Design review of the part built by this model. Coordinates are the model's own, in mm. A direction names the side the tool comes from. Round coordinates to 2 decimals unless told otherwise and drop trailing zeros. Order: outer loops, then holes, each group sorted by start corner. A loop starts at its lowest first (then second) coordinate and runs counter-clockwise, first axis right, second up. Notation, with made-up numbers: M 69,47 L 76,47 A10 cw 76,65 Z; hole C 88.25,83.25 d11. An arc over 180 degrees is marked long. Write each question's results on one line, items separated by ' | '. Start each with the question number.
Item 1: Take a section at B-B, the plane x = 14. Write out the cut boundary in (y, z), plus the area to 3 significant figures.
Item 2: The part is to be moulded in two halves that separate along Z. For faces 1 (the cylindrical face through (-38.356, 14.529, -14.345)), 2 (the cylindrical face through (101.339, -33.056, -8.385)), 3 (the flat face through (-23, 8, -18.019)), 4 (the flat face through (25, -3, 0)), say which applies: +Z half, -Z half, draft (parallel to the pull), parting line (faces both ways), or undercut.
Item 3: Take a section at A-A, the plane z = 3.5. Write out the cut boundary in (x, y).
Item 4: Machinability: for faces 5 (the flat face through (94.126, -28.892, -9.07)), 6 (the flat face through (24, -4.5, -9)), 7 (the flat face through (79.126, -20.232, -8.93)), which of the approach directions +Z, -Z, +X, -X, +Y, -Y give a long, thin tool a straight path to every point of the face, cutting with its end or side? Answer none if there is none.
Item 5: Clearance check with flat-ended pins moving along their axes: pin 1 (0.6 mm diameter, centred on x = 27, z = -16.5, fed in from +Y); pin 2 (10 mm diameter, centred on y = -12.5, z = 1.5, fed in from -X); pin 3 (7 mm diameter, centred on x = 22.5, z = -8.5, fed in from +Y); pin 4 (9 mm diameter, centred on x = 12, y = -12, fed in from -Z). State where each tip first meets the part, or that it passes through.
Item 6: Wall thickness on line 1 (Z direction, x = -11.5, y = 3); line 2 (Y direction, x = 45.5, z = -4); line 3 (X direction, y = 7, z = -15): over which ranges is each line inside the solid? List them lowest first. Write a range as [from, to].
Item 7: Take a section at C-C, the plane y = -7.5. Write out the cut boundary in (x, z).
```python
from build123d import *

# Parameters (mm, degrees)
EXTRUDE_START       = 1.5
EXTRUDE_1_DEPTH     = 6
FILLET_1_R          = 1
FILLET_2_R          = 5
FILLET_3_R          = 3
CUT_EXTRUDE_1_DEPTH = 1.5
FILLET_4_R          = 2
CUT_EXTRUDE_START   = -4.5
CUT_EXTRUDE_2_DEPTH = 1.5
FILLET_5_R          = 2
EXTRUDE_2_DEPTH     = 6
CUT_EXTRUDE_3_DEPTH = 1.5
FILLET_6_R          = 2
CUT_EXTRUDE_4_DEPTH = 1.5
FILLET_7_R          = 2


with BuildPart() as part:
    # 扫描2: sweep along a path in 草图1
    with BuildLine(Plane.XY) as sweep_2_path:
        Line((-19.938771315, 9.297601758), (0, 0))
        Line((0, 0), (50, 0))
        Line((50, 0), (69.052558883, -11))
    # 草图2 → 扫描2 (sweep)
    with BuildSketch(Plane(origin=(0, 0, 0), x_dir=(0, 0, -1), z_dir=(1, 0, 0))):
        Polygon((0, 0), (2, 0), (2, -1.5), (16, -1.5), (16, 0), (18, 0), (18, -6), (16, -6), (16, -4.5), (2, -4.5), (2, -6), (0, -6), align=None)
    sweep(path=sweep_2_path.line, transition=Transition.RIGHT)

    # 草图3 → 凸台-拉伸1 (add)
    with BuildSketch(Plane(origin=(-0.633927393, -1.359461681, 0), x_dir=(0.9063077870366528, -0.42261826174069356, 0), z_dir=(0.42261826174069356, 0.9063077870366528, 0)).offset(EXTRUDE_START)):
        with BuildLine():
            Line((-22, 9), (-22, 18.019216451))
            Line((-22, 18.019216451), (-29.589804491, 18.019216451))
            ThreePointArc((-29.589804491, 18.019216451), (-45.578071203, 25.926597156), (-59.82908715, 15.2))
            Line((-59.82908715, 15.2), (-40, 15.2))
            Line((-40, 15.2), (-40, 9))
            Line((-40, 9), (-40, 2.8))
            Line((-40, 2.8), (-59.82908715, 2.8))
            ThreePointArc((-59.82908715, 2.8), (-45.56678948, -7.927645162), (-29.577794898, 0))
            Line((-29.577794898, 0), (-22, 0))
            Line((-22, 0), (-22, 9))
        make_face()
    extrude(amount=-EXTRUDE_1_DEPTH)

    # 圆角1
    fillet_1_edges = [part.edges().sort_by_distance(p)[0] for p in [
        (-55.49142236, 22.565941452, -2.8),
        (-55.49142236, 22.565941452, -15.2),
    ]]
    fillet(fillet_1_edges, radius=FILLET_1_R)

    # 圆角2
    fillet_2_edges = [part.edges().sort_by_distance(p)[0] for p in [
        (-28.085325012, 9.786268378, -18.019216451),
        (-28.074440625, 9.781192905, 0),
    ]]
    fillet(fillet_2_edges, radius=FILLET_2_R)

    # 圆角3
    fillet_3_edges = [part.edges().sort_by_distance(p)[0] for p in [
        (-37.520166267, 14.185807109, -2.8),
        (-37.520166267, 14.185807109, -15.2),
    ]]
    fillet(fillet_3_edges, radius=FILLET_3_R)

    # 草图4 → 切除-拉伸1 (cut)
    with BuildSketch(Plane(origin=(0, 0, 0), x_dir=(0.9063077870366528, -0.42261826174069356, 0), z_dir=(0.42261826174069356, 0.9063077870366528, 0))):
        with BuildLine():
            Line((-22, 16), (-28.508066615, 16))
            ThreePointArc((-28.508066615, 16), (-27, 9), (-28.508066615, 2))
            Line((-28.508066615, 2), (-22, 2))
            Line((-22, 2), (-22, 16))
        make_face()
    extrude(amount=-CUT_EXTRUDE_1_DEPTH, mode=Mode.SUBTRACT)

    # 圆角4
    fillet_4_edges = [part.edges().sort_by_distance(p)[0] for p in [
        (-26.154046463, 11.368298718, -2),
        (-26.154046463, 11.368298718, -16),
    ]]
    fillet(fillet_4_edges, radius=FILLET_4_R)

    # 草图4<2> → 切除-拉伸2 (cut)
    with BuildSketch(Plane(origin=(0, 0, 0), x_dir=(0.9063077870366528, -0.42261826174069356, 0), z_dir=(0.42261826174069356, 0.9063077870366528, 0)).offset(CUT_EXTRUDE_START)):
        with BuildLine():
            Line((-22, 16), (-28.508066615, 16))
            ThreePointArc((-28.508066615, 16), (-27, 9), (-28.508066615, 2))
            Line((-28.508066615, 2), (-22, 2))
            Line((-22, 2), (-22, 16))
        make_face()
    extrude(amount=-CUT_EXTRUDE_2_DEPTH, mode=Mode.SUBTRACT)

    # 圆角5
    fillet_5_edges = [part.edges().sort_by_distance(p)[0] for p in [
        (-28.055828641, 7.289913677, -16),
        (-28.055828641, 7.289913677, -2),
    ]]
    fillet(fillet_5_edges, radius=FILLET_5_R)

    # 草图7 → 凸台-拉伸2 (add)
    with BuildSketch(Plane(origin=(12.5, 21.650635095, 0), x_dir=(0.866025403784438, -0.5000000000000012, 0), z_dir=(0.5000000000000011, 0.8660254037844379, 0))):
        with BuildLine():
            Line((72.879065087, 18), (65.301270189, 18))
            Line((65.301270189, 18), (65.301270189, 16))
            Line((65.301270189, 16), (65.301270189, 0))
            Line((65.301270189, 0), (72.879065087, 0))
            ThreePointArc((72.879065087, 0), (104.301270189, 9), (72.879065087, 18))
        make_face()
        Polygon((78.641016151, 14), (87.301270189, 19), (95.961524227, 14), (95.961524227, 4), (87.301270189, -1), (78.641016151, 4), align=None, mode=Mode.SUBTRACT)
    extrude(amount=-EXTRUDE_2_DEPTH)

    # 草图8 → 切除-拉伸3 (cut)
    with BuildSketch(Plane(origin=(12.5, 21.650635095, 0), x_dir=(0.866025403784438, -0.5000000000000012, 0), z_dir=(0.5000000000000011, 0.8660254037844379, 0))):
        with BuildLine():
            Line((65.301270189, 16), (65.301270189, 2))
            Line((65.301270189, 2), (71.809336804, 2))
            ThreePointArc((71.809336804, 2), (70.301270189, 9), (71.809336804, 16))
            Line((71.809336804, 16), (65.301270189, 16))
        make_face()
    extrude(amount=-CUT_EXTRUDE_3_DEPTH, mode=Mode.SUBTRACT)

    # 圆角6
    fillet_6_edges = [part.edges().sort_by_distance(p)[0] for p in [
        (74.313709902, -14.90355236, -16),
        (74.313709902, -14.90355236, -2),
    ]]
    fillet(fillet_6_edges, radius=FILLET_6_R)

    # 草图8<2> → 切除-拉伸4 (cut)
    with BuildSketch(Plane(origin=(12.5, 21.650635095, 0), x_dir=(0.866025403784438, -0.5000000000000012, 0), z_dir=(0.5000000000000011, 0.8660254037844379, 0)).offset(CUT_EXTRUDE_START)):
        with BuildLine():
            Line((65.301270189, 16), (65.301270189, 2))
            Line((65.301270189, 2), (71.809336804, 2))
            ThreePointArc((71.809336804, 2), (70.301270189, 9), (71.809336804, 16))
            Line((71.809336804, 16), (65.301270189, 16))
        make_face()
    extrude(amount=-CUT_EXTRUDE_4_DEPTH, mode=Mode.SUBTRACT)

    # 圆角7
    fillet_7_edges = [part.edges().sort_by_distance(p)[0] for p in [
        (72.063709902, -18.800666677, -16),
        (72.063709902, -18.800666677, -2),
    ]]
    fillet(fillet_7_edges, radius=FILLET_7_R)


solid = part.part
```
Results list:
1) outline: M -6,-18 L 0,-18 L 0,-16 L -1.5,-16 L -1.5,-2 L 0,-2 L 0,0 L -6,0 L -6,-2 L -4.5,-2 L -4.5,-16 L -6,-16 Z | area: 66.0 mm²
2) face 1: undercut | face 2: parting line | face 3: -Z half | face 4: +Z half
3) outline: M -52.86,18.03 L -31.97,8.29 L -29.44,13.73 L -50.32,23.46 Z; M 75.13,-21.44 L 95.08,-32.96 L 98.08,-27.76 L 78.13,-16.24 Z
4) face 5: -X, +Y | face 6: -X, -Y | face 7: +X, -Y
5) pin 1: y = 0 | pin 2: x = 51.39 | pin 3: y = -1.5 | pin 4: through
6) line 1: [-18, 0] | line 2: [-4.5, -1.5] | line 3: [-29.21, -26.97], [-25.66, -18.56]
7) outline: M 50.99,-18 L 62.99,-18 L 62.99,-16 L 59.99,-16 L 59.99,-2 L 62.99,-2 L 62.99,0 L 50.99,0 L 50.99,-2 L 53.99,-2 L 53.99,-16 L 50.99,-16 Z
